```python
from build123d import *

# Parameters (mm, degrees)
BOSS_EXTRUDE1_DEPTH = 12
SKETCH1_3_W         = 12
SKETCH1_3_H         = 8
BOSS_EXTRUDE2_DEPTH = 25
SKETCH2_R           = 4.5
CUT_EXTRUDE1_DEPTH  = 8
SKETCH4_R           = 2.5
CUT_EXTRUDE2_DEPTH  = 8


with BuildPart() as part:
    # Sketch1 → Boss-Extrude1 (new body)
    with BuildSketch(Plane(origin=(0, 0, 0), x_dir=(0, 0, -1), z_dir=(1, 0, 0))):
        Polygon((0, 0), (125.37946203, 0), (135.304113157, 5.73), (154.39, 5.73), (154.39, 13.73), (135.304113157, 13.73), (125.37946203, 8), (0, 8), align=None)
    extrude(amount=-BOSS_EXTRUDE1_DEPTH)

    # Sketch1<3> → Boss-Extrude2 (add)
    with BuildSketch(Plane(origin=(0, 0, 0), x_dir=(0, 0, -1), z_dir=(1, 0, 0))):
        with Locations((6, 4)):
            Rectangle(SKETCH1_3_W, SKETCH1_3_H)
    extrude(amount=-BOSS_EXTRUDE2_DEPTH)

    # Sketch2 → Cut-Extrude1 (cut)
    with BuildSketch(Plane(origin=(0, 8, 0), x_dir=(1, 0, 0), z_dir=(0, 1, 0))):
        with Locations(Location((-16.59, 6, 0), (0, 0, 270))):
            Circle(SKETCH2_R)
    extrude(amount=-CUT_EXTRUDE1_DEPTH, mode=Mode.SUBTRACT)

    # Sketch4 → Cut-Extrude2 (cut)
    with BuildSketch(Plane(origin=(0, 13.73, 0), x_dir=(1, 0, 0), z_dir=(0, 1, 0))):
        with Locations(Location((-6, 144.02, 0), (0, 0, 270))):
            Circle(SKETCH4_R)
    extrude(amount=-CUT_EXTRUDE2_DEPTH, mode=Mode.SUBTRACT)


solid = part.part
```
For this review, take the finished solid that the model builds, in its own axes (mm). A direction names the side the tool comes from. Give positions to 0.01 mm unless a question says otherwise; leave off trailing zeros. Write each loop counter-clockwise with the first axis right and the second up, starting at its lowest first coordinate (ties: lowest second). Pieces come first, ordered by that corner, then holes. Notation, with made-up numbers: M -9.75,-12 L 36.25,-12 A25 ccw 36.25,2 Z; hole C 25,-6.5 d4. An arc over 180 degrees is marked long. Answer as a JSON object with one key per item and string values. Group by question number.
Item 1: Consider section C-C on x = -10.5. Write out the cut boundary in (y, z).
Item 2: Consider section A-A on x = -16.59. Write out the cut boundary in (y, z), plus the area to 3 significant figures.
Item 3: For pin 1 Ø4 at (x, z) = (-6, -144.02) entering from +Y; pin 2 Ø2.5 at (x, y) = (-19, 3) entering from -Z; pin 3 Ø3 at (y, z) = (3, -132.5) entering from -X; pin 4 Ø13 at (x, z) = (-3, -148.5) entering from -Y, all flat-tipped, find the tip position at first contact; note any pin that passes through.
Item 4: For probe 1 along X at (y, z) = (4.5, -6); probe 2 along Z at (x, y) = (-16.5, 1.75); probe 3 along X at (y, z) = (8.75, -144.02), list the stretches that pass through material, from the lowest coordinate up. Write a range as [from, to].
Item 5: Tool access review of faces 4 (the flat face through (-7, 8, -64)), 5 (the flat face through (-12, 5, -82)), 6 (the flat face through (-6, 5.73, -147)): name each direction out of +Z, -Z, +X, -X, +Y, -Y from which nothing blocks a thin tool from reaching the whole face with its end or side.
Item 6: Consider section D-D on y = 10.25. Write out the cut boundary in (x, z).
Item 7: Draft analysis for pull direction Z (two halves, no side actions). For faces 1 (the flat face through (-6, 10, -154.39)), 2 (the flat face through (-25, 4, -6)), 3 (the cylindrical face through (-5.89, 9.786, -146.518)), state which applies: +Z half, -Z half, draft (parallel to the pull), parting line (faces both ways), or undercut.
Item 8: Consider section B-B on z = -144.02. Write out the cut boundary in (x, y).
Check result:
{
 "1": {"outline": "M 0,-125.38 L 5.73,-135.3 L 5.73,-154.39 L 13.73,-154.39 L 13.73,-135.3 L 8,-125.38 L 8,0 L 0,0 Z"},
 "2": {"outline": "M 0,-12 L 8,-12 L 8,-10.5 L 0,-10.5 Z; M 0,-1.5 L 8,-1.5 L 8,0 L 0,0 Z", "area": "24.0 mm^2"},
 "3": {"pin 1": "passes through", "pin 2": "stops at z = -12", "pin 3": "stops at x = -12", "pin 4": "stops at y = 5.73"},
 "4": {"probe 1": "x = [-25, -21.09], [-12.09, 0]", "probe 2": "z = [-12, -10.5], [-1.5, 0]", "probe 3": "x = [-12, -8.5], [-3.5, 0]"},
 "5": {"face 4": "+Z, +X, -X, +Y", "face 5": "-Z, -X, +Y, -Y", "face 6": "-Z, +X, -X, -Y"},
 "6": {"outline": "M -12,-154.39 L 0,-154.39 L 0,-129.28 L -12,-129.28 Z; hole C -6,-144.02 d5"},
 "7": {"face 1": "-Z half", "face 2": "draft", "face 3": "undercut"},
 "8": {"outline": "M -12,5.73 L -8.5,5.73 L -8.5,13.73 L -12,13.73 Z; M -3.5,5.73 L 0,5.73 L 0,13.73 L -3.5,13.73 Z"}
}
